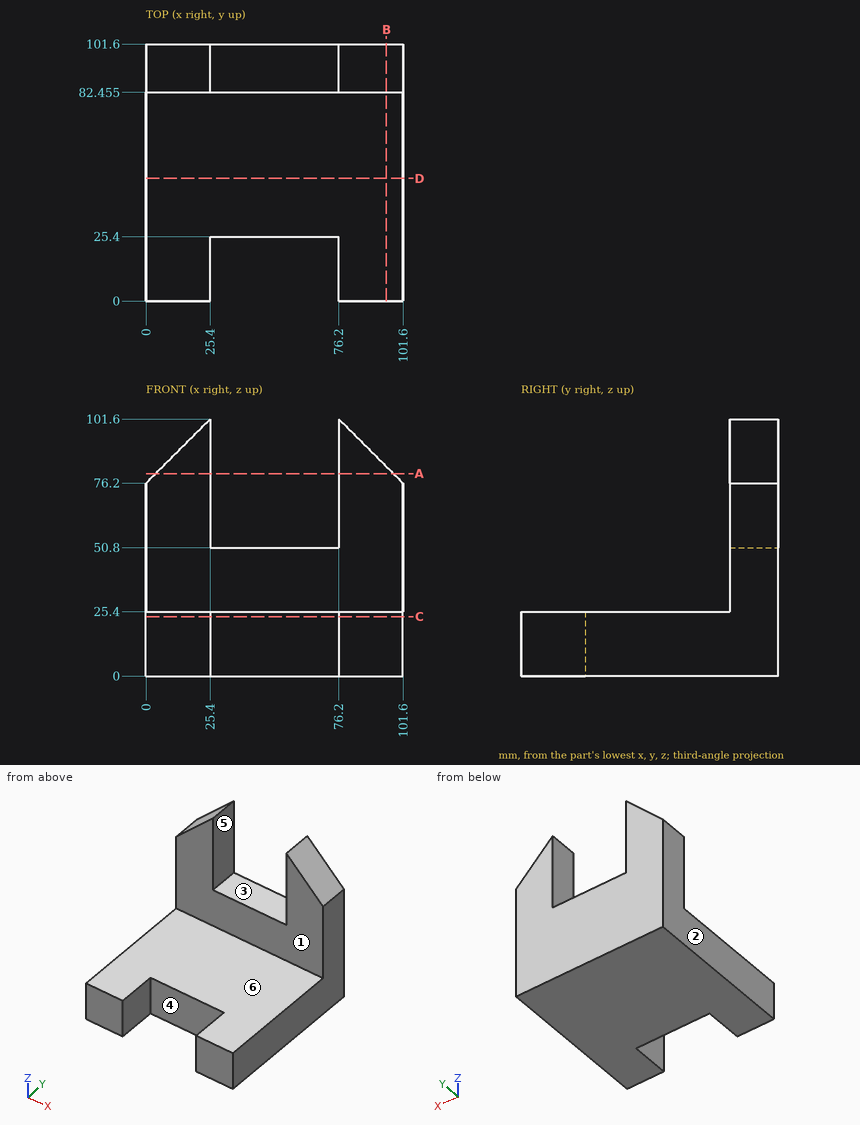
Geometry: see drawing. Coordinates: mm, zero at the bounding-box minimum. A direction names the side the tool comes from. Coordinates: 2 decimals unless noted, no trailing zeros. Order: outer loops, then holes, each group sorted by start corner. A loop starts at its lowest first (then second) coordinate and runs counter-clockwise, first axis right, second up. Notation, with made-up numbers: (19.25, -4) - (66.25, -4) arc R38 ccw to (66.25, 35) - close; hole circle Ø1 at (-36.5, 89). An arc over 180 degrees is marked (long way). Use one line per item in the form item = value.
1) Section B-B (x = 95). Return loops of the section in (y, z) (3 decimals), then the cut area to 3 significant figures.
Solutions:
outline = (0, 0) - (101.6, 0) - (101.6, 82.8) - (82.455, 82.8) - (82.455, 25.4) - (0, 25.4) - close
area = 3,680 mm^2
2) Section C-C (z = 23.5). Return loops of the section in (x, y).
Solutions:
outline = (0, 0) - (25.4, 0) - (25.4, 25.4) - (76.2, 25.4) - (76.2, 0) - (101.6, 0) - (101.6, 101.6) - (0, 101.6) - close
3) Section D-D (y = 48.5). Return loops of the section in (x, z).
Solutions:
outline = (0, 0) - (101.6, 0) - (101.6, 25.4) - (0, 25.4) - close
4) Set-up query: the marked faces 4, 5 and 6. Return all of +Z, -Z, +X, -X, +Y, -Y with unobstructed straight access to the full face (end or side cutting, diameter ignored); none if empty.
Solutions:
face_4 = +Z, -Z, -Y
face_5 = +Z, +Y, -Y
face_6 = +Z, +X, -X, -Y
5) Pin query (flat end, axial travel): pin 1 (21 mm diameter, centred on x = 59.5, y = 93.5, fed in from +Z); pin 2 (23 mm diameter, centred on x = 50, z = 46, fed in from -Y) (3 decimals); pin 3 (24.5 mm diameter, centred on x = 50.5, y = 25, fed in from +Z). Return the tip coordinate at first contact, or that it passes through.
Solutions:
pin_1 = 50.8
pin_2 = 82.455
pin_3 = 25.4
6) Section A-A (z = 80). Return loops of the section in (x, y) (3 decimals), then the cut area to 3 significant figures.
Solutions:
outline = (3.8, 82.455) - (25.4, 82.455) - (25.4, 101.6) - (3.8, 101.6) - close; (76.2, 82.455) - (97.8, 82.455) - (97.8, 101.6) - (76.2, 101.6) - close
area = 827 mm^2
7) Ray query, L1, parallel to X at y = 20.5, z = 15; L2, parallel to Z at x = 24.5, y = 25.5; L3, parallel to Y at x = 18.5, z = 31 (3 decimals). Return the intervals inside material, ascending.
Solutions:
L1 = 0 to 25.4, 76.2 to 101.6
L2 = 0 to 25.4
L3 = 82.455 to 101.6
8) Mould query, pull axis X, two halves, no side actions, for the marked faces 1, 2 and 3. Classes: +X half, -X half, draft (parallel to the pull), parting line (faces both ways), or undercut.
Solutions:
face_1 = draft
face_2 = -X half
face_3 = undercut
